Verification items for the finished model (mm, model axes). Face numbers are marked on the shaded views. A direction names the side the tool comes from. Give positions to 0.01 mm unless a question says otherwise; leave off trailing zeros. Loops run counter-clockwise (first coordinate to the right, second up) from the corner with the lowest first, then second, coordinate; pieces in that order, holes last. Notation, with made-up numbers: (8.25, 8) - (50.25, 8) arc R14 cw to (50.25, 24) - close; hole circle Ø7 at (-15, 64). An arc over 180 degrees is marked (long way). One line per question, with ' | ' between items. Start each with the question number.
1. Thickness scan on line 1 along X through (y, z) = (28.5, 7); line 2 along Z through (x, y) = (8, 33.5); line 3 along X through (y, z) = (5.5, 110.5). Record the ranges inside material, lowest first. Write a range as from..to.
2. Mould release check, pull along Z, two halves, no side actions. Record for the marked faces 1, 2, 3 and 4: +Z half, -Z half, draft (parallel to the pull), parting line (faces both ways), or undercut.
3. Section check B-B, the plane x = 12. Enter the section's corners in (y, z).
4. Section check D-D, the plane y = 41.5. Enter the section's corners in (x, z), then the cut area to 3 significant figures.
5. Section check A-A, the plane z = 62.5. Enter the section's corners in (x, y).
6. Section check C-C, the plane y = 25. Enter the section's corners in (x, z), then the cut area to 3 significant figures.
7. Depth check by flat-ended pin: pin 1 Ø5 at (y, z) = (10, 37.5) entering from +X; pin 2 Ø5 at (y, z) = (41.5, 64.5) entering from +X; pin 3 Ø6 at (y, z) = (27.5, 16.5) entering from +X; pin 4 Ø10 at (x, y) = (-12.5, 28.5) entering from -Z. Enter the tip coordinate at first touch or a pass-through.
8. Tool access check on the marked faces 5, 6 and 7. Record the directions out of +Z, -Z, +X, -X, +Y, -Y that give a thin tool (end or side, any length) a straight path to the whole face; none if there is none.
from build123d import *

# Parameters (mm, degrees)
SKETCH1_W           = 31
SKETCH1_H           = 120
SKETCH1_W_2         = 21
SKETCH1_H_2         = 110
BOSS_EXTRUDE4_DEPTH = 48
SKETCH6_W           = 20
SKETCH6_H           = 20
CUT_EXTRUDE3_DEPTH  = 136
BOSS_EXTRUDE5_DEPTH = 120


with BuildPart() as part:
    # Sketch1 → Boss-Extrude4 (new body)
    with BuildSketch(Plane(origin=(0, 0, 0), x_dir=(1, 0, 0), z_dir=(0, 1, 0))):
        with Locations((8.759280296, -55.007974482)):
            Rectangle(SKETCH1_W, SKETCH1_H)
        with Locations((8.759280296, -55.007974482)):
            Rectangle(SKETCH1_W_2, SKETCH1_H_2, mode=Mode.SUBTRACT)
    extrude(amount=BOSS_EXTRUDE4_DEPTH)

    # Sketch6 → Cut-Extrude3 (cut)
    with BuildSketch(Plane.XY.offset(115.007974482)):
        with Locations((8.759280296, 10)):
            Rectangle(SKETCH6_W, SKETCH6_H)
    extrude(amount=-CUT_EXTRUDE3_DEPTH, mode=Mode.SUBTRACT)

    # Sketch7 → Boss-Extrude5 (add)
    with BuildSketch(Plane.XY.offset(115.007974482)):
        Polygon((-6.740719704, 38.947441117), (-11.967217013, 48), (-17.740719704, 48), (-6.740719704, 28.947441117), align=None)
        Polygon((24.259280296, 38.947441117), (24.259280296, 28.947441117), (35.259280296, 48), (29.485777604, 48), align=None)
    extrude(amount=-BOSS_EXTRUDE5_DEPTH)


solid = part.part
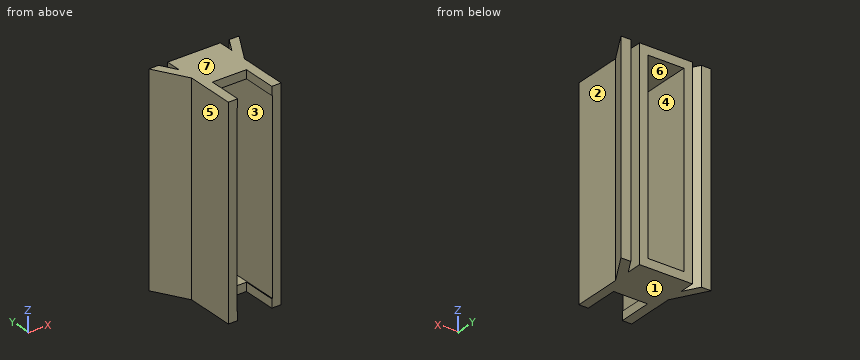
Results list:
1) line 1: -6.74..-1.74, 19.26..24.26 | line 2: -4.99..0.01, 110.01..115.01 | line 3: -6.74..-1.24, 18.76..24.26
2) face 1: -Z half | face 2: draft | face 3: undercut | face 4: undercut
3) outline: (20, -4.99) - (48, -4.99) - (48, 0.01) - (20, 0.01) - close; (20, 110.01) - (48, 110.01) - (48, 115.01) - (20, 115.01) - close
4) outline: (-13.99, -4.99) - (-8.21, -4.99) - (-8.21, 115.01) - (-13.99, 115.01) - close; (-6.74, -4.99) - (24.26, -4.99) - (24.26, 115.01) - (-6.74, 115.01) - close; (25.73, -4.99) - (31.51, -4.99) - (31.51, 115.01) - (25.73, 115.01) - close; hole (-1.74, 0.01) - (19.26, 0.01) - (19.26, 110.01) - (-1.74, 110.01) - close | area: 2,800 mm²
5) outline: (-17.74, 48) - (-6.74, 28.95) - (-6.74, 0) - (-1.74, 0) - (-1.74, 48) - (-6.74, 48) - (-6.74, 38.95) - (-11.97, 48) - close; (19.26, 0) - (24.26, 0) - (24.26, 28.95) - (35.26, 48) - (29.49, 48) - (24.26, 38.95) - (24.26, 48) - (19.26, 48) - close
6) outline: (-6.74, -4.99) - (24.26, -4.99) - (24.26, 115.01) - (-6.74, 115.01) - close; hole (-1.74, 0.01) - (19.26, 0.01) - (19.26, 110.01) - (-1.74, 110.01) - close | area: 1,410 mm²
7) pin 1: x = 24.26 | pin 2: x = 32.95 | pin 3: x = 25.16 | pin 4: through
8) face 5: +Z, -Z, -X, -Y | face 6: +Y, -Y | face 7: +Z, +X, -X, +Y, -Y
